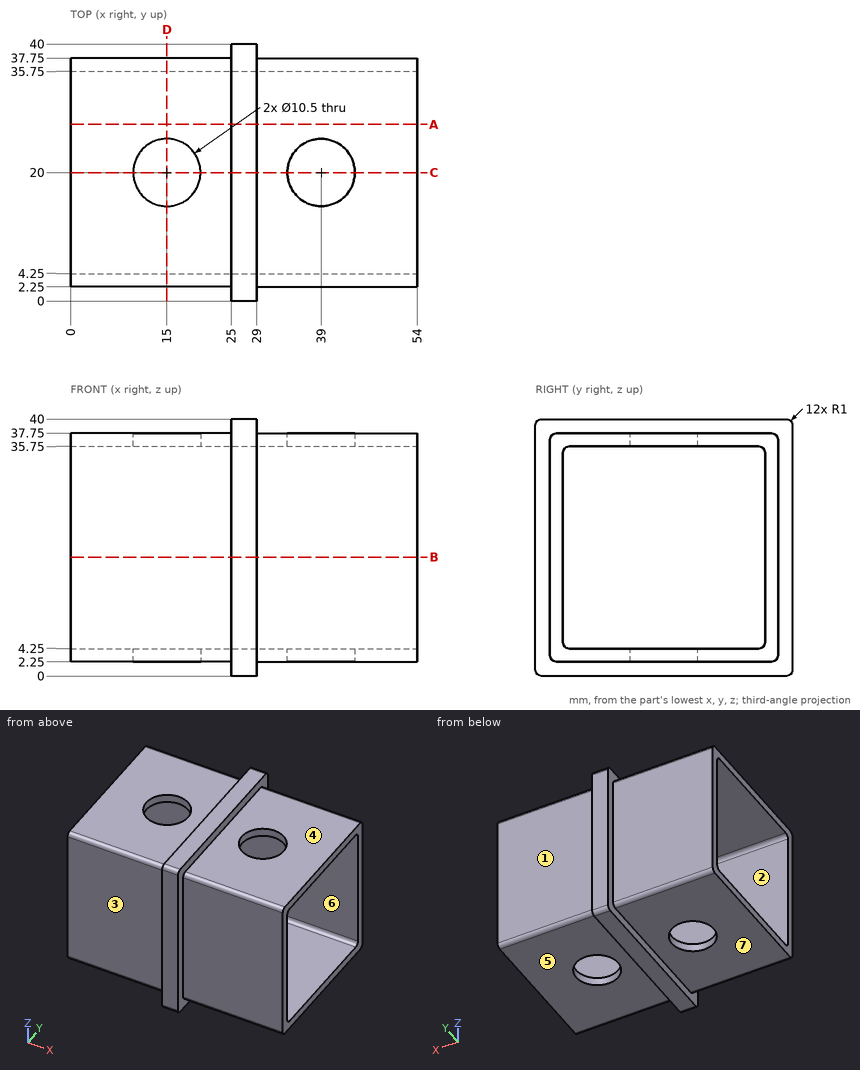
Could you check a few things on this drawing? It's one solid part, dimensions in mm from its lowest x, y, z. A direction names the side the tool comes from. Coordinates: 2 decimals unless noted, no trailing zeros. Order: outer loops, then holes, each group sorted by start corner. A loop starts at its lowest first (then second) coordinate and runs counter-clockwise, first axis right, second up. Notation, with made-up numbers: M 32.25,29 L 73.25,29 A4 ccw 73.25,34 Z; hole C 15.25,-25.75 d6. An arc over 180 degrees is marked long. Use one line per item in the form item = value. Start each with the question number.
1. Suppose I cut it at C-C on y = 20. Count the separate pieces of the cut face and the enclosed holes in it, then the cut area to 3 significant figures.
2. On a 3-axis mill with a long thin cutter (end or side, diameter ignored), from which of +Z, -Z, +X, -X, +Y, -Y can I reach the whole of each face in a straight line? I mean the marked faces 4, 5, 6 and 7. Say none if no direction works.
3. We'd pull the mould along Y, two halves only. Please class the marked faces 1, 2 and 3: +Y half, -Y half, draft (parallel to the pull), parting line (faces both ways), or undercut.
4. Suppose I cut it at D-D on x = 15. Write out the boundary of the cut face in (y, z).
5. Please list where these lines run through material, in increasing order: line 1 (Y direction, x = 42.5, z = 23.5); line 2 (Y direction, x = 39, z = 3.75).
6. For pin 1 (12 mm diameter, centred on x = 39, z = 31, fed in from +Y); pin 2 (12.5 mm diameter, centred on x = 13, y = 19, fed in from -Z); pin 3 (12 mm diameter, centred on x = 15, y = 20, fed in from +Z); pin 4 (8 mm diameter, centred on y = 32.5, z = 28.5, fed in from +X), each with a flat end and sliding along its axis, tell me the tip position at first contact or that it passes through.
7. Suppose I cut it at A-A on y = 27.5. Write out the boundary of the cut face in (x, z).
Geometry says:
q1.separate_pieces = 6
q1.enclosed_holes = 0
q1.area = 150 mm^2
q2.face_4 = +Z, +X, +Y, -Y
q2.face_5 = -Z, +X, +Y, -Y
q2.face_6 = +X, -X
q2.face_7 = -Z, -X, +Y, -Y
q3.face_1 = +Y half
q3.face_2 = undercut
q3.face_3 = -Y half
q4.outline = M 2.25,3.25 A1 ccw 3.25,2.25 L 14.75,2.25 L 14.75,4.25 L 5.25,4.25 A1 cw 4.25,5.25 L 4.25,34.75 A1 cw 5.25,35.75 L 14.75,35.75 L 14.75,37.75 L 3.25,37.75 A1 ccw 2.25,36.75 Z; M 25.25,2.25 L 36.75,2.25 A1 ccw 37.75,3.25 L 37.75,36.75 A1 ccw 36.75,37.75 L 25.25,37.75 L 25.25,35.75 L 34.75,35.75 A1 cw 35.75,34.75 L 35.75,5.25 A1 cw 34.75,4.25 L 25.25,4.25 Z
q5.line_1 = 2.25 to 4.25, 35.75 to 37.75
q5.line_2 = 2.25 to 14.75, 25.25 to 37.75
q6.pin_1 = 37.75
q6.pin_2 = 2.25
q6.pin_3 = 37.75
q6.pin_4 = 54
q7.outline = M 0,2.25 L 25,2.25 L 25,0 L 29,0 L 29,2.25 L 54,2.25 L 54,4.25 L 0,4.25 Z; M 0,35.75 L 54,35.75 L 54,37.75 L 29,37.75 L 29,40 L 25,40 L 25,37.75 L 0,37.75 Z
